Autodesk Inventor part; units mm, degrees
ref_plane "YZ Plane" through (0, 0, 0) normal (1, 0, 0) x (0, 1, 0)
ref_plane "XZ Plane" through (0, 0, 0) normal (0, 1, 0) x (-1, 0, 0)
ref_plane "XY Plane" through (0, 0, 0) normal (0, 0, 1) x (1, 0, 0)
sketch "Sketch1" plane through (0, 0, 0) normal (0, 1, 0) x (-1, 0, 0)
  circle A0 centre (0, 0) radius 11.4
  dimension "d2" = 22.8
extrude "Extrusion1" add sketch "Sketch1" along normal blind 60
sketch "Sketch2" plane through (0, 60, 0) normal (0, 1, 0) x (1, 0, 0)
  circle A0 centre (0, 0) radius 8.75
  dimension "d3" = 17.5
extrude "Extrusion2" add sketch "Sketch2" along normal blind 10
fillet "Fillet1" radius 1.5 1 edges at (11.4, 60, 0)
thread "Thread1"
sketch "Sketch3" plane through (0, 70, 0) normal (0, 1, 0) x (1, 0, 0)
  circle A0 centre (0, 0) radius 5.625
  dimension "d9" = 11.25
extrude "Extrusion3" cut sketch "Sketch3" against normal blind 65
fillet "Fillet2" radius 1 2 edges at (11.4, 0, 0) (-8.75, 70, 0)
sketch "Sketch4" plane through (0, 5, 0) normal (0, 1, 0) x (1, 0, 0)
  circle A0 centre (0, 0) radius 9
  dimension "d13" = 18
extrude "Extrusion4" cut sketch "Sketch4" along normal blind 50
properties part number "Vial"
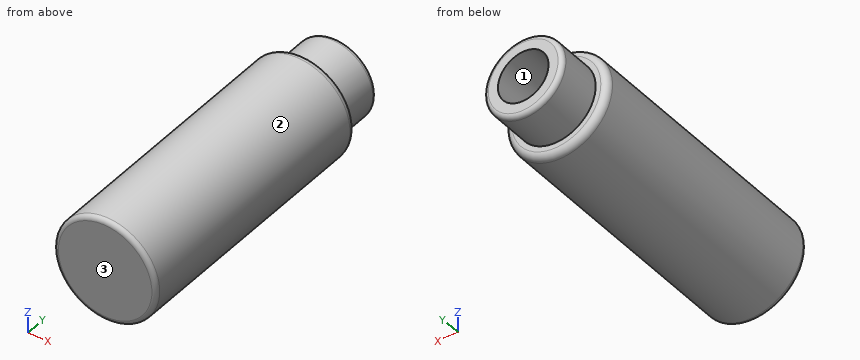
Geometry: final body of the model. Coordinates: model frame, mm. Face numbers are marked on the shaded views. Round coordinates to 2 decimals unless told otherwise and drop trailing zeros. Loops run counter-clockwise (first coordinate to the right, second up) from the corner with the lowest first, then second, coordinate; pieces in that order, holes last.
Q1. Material intervals for L1, parallel to Y at x = 3.75, z = -5; L2, parallel to Z at x = 0, y = 31.5; L3, parallel to X at y = 62.75, z = 0 (3 decimals), sorted ascending.
Q2. Section B-B on x = 0. Return loops of the section in (y, z) (3 decimals).
Q3. Pin query (flat end, axial travel): P1, Ø2, axis at y = 56.5, z = 1, coming from the +X side; P2, Ø11, axis at x = 0, z = 0, coming from the +Y side; P3, Ø8, axis at y = 62, z = -6.5, coming from the +X side; P4, Ø8, axis at x = -8, y = 38.5, coming from the +Z side. Return the tip coordinate at first contact, or that it passes through.
Q4. Section C-C on y = 40. Return loops of the section in (x, z), plus the area to 3 significant figures.
Q5. Pull-direction query (X, two-part tool) for the marked faces 1, 2 and 3; classes: released by +X, released by -X, zero draft, split by the parting line, or undercut.
Q6. Section A-A on z = 0. Return loops of the section in (x, y) (3 decimals), plus the area to 3 significant figures.
Evaluation:
1. L1: y = 0 to 5, 55 to 70
1. L2: z = -11.4 to -9, 9 to 11.4
1. L3: x = -8.75 to -5.625, 5.625 to 8.75
2. outline: (0, -10.4) arc R1 ccw to (1, -11.4) - (58.5, -11.4) arc R1.5 ccw to (60, -9.9) - (60, -8.75) - (69, -8.75) arc R1 ccw to (70, -7.75) - (70, -5.625) - (55, -5.625) - (55, -9) - (5, -9) - (5, 9) - (55, 9) - (55, 5.625) - (70, 5.625) - (70, 7.75) arc R1 ccw to (69, 8.75) - (60, 8.75) - (60, 9.9) arc R1.5 ccw to (58.5, 11.4) - (1, 11.4) arc R1 ccw to (0, 10.4) - close
3. P1: stops at x = 11.4
3. P2: stops at y = 5
3. P3: stops at x = 10.64
3. P4: stops at z = 10.68
4. outline: circle Ø22.8 at (0, 0); hole circle Ø18 at (0, 0)
4. area: 154 mm2
5. face 1: undercut
5. face 2: split by the parting line
5. face 3: zero draft
6. outline: (-11.4, 1) arc R1 ccw to (-10.4, 0) - (10.4, 0) arc R1 ccw to (11.4, 1) - (11.4, 58.5) arc R1.5 ccw to (9.9, 60) - (8.75, 60) - (8.75, 69) arc R1 ccw to (7.75, 70) - (5.625, 70) - (5.625, 55) - (9, 55) - (9, 5) - (-9, 5) - (-9, 55) - (-5.625, 55) - (-5.625, 70) - (-7.75, 70) arc R1 ccw to (-8.75, 69) - (-8.75, 60) - (-9.9, 60) arc R1.5 ccw to (-11.4, 58.5) - close
6. area: 472 mm2
